from build123d import *

# Parameters (mm, degrees)
CROQUIS1_W              = 130
CROQUIS1_H              = 130
SALIENTE_EXTRUIR1_DEPTH = 60
REDONDEO1_R             = 10
VACIADO1_T              = -4
CORTAR_EXTRUIR1_START   = -58
CORTAR_EXTRUIR1_DEPTH   = 1
CORTAR_EXTRUIR2_START   = -56
CORTAR_EXTRUIR2_DEPTH   = 1
CORTAR_EXTRUIR3_START   = -4
CORTAR_EXTRUIR3_DEPTH   = 1


with BuildPart() as part:
    # Croquis1 → Saliente-Extruir1 (new body)
    with BuildSketch(Plane(origin=(0, 0, 0), x_dir=(1, 0, 0), z_dir=(0, 1, 0))):
        Rectangle(CROQUIS1_W, CROQUIS1_H)
    extrude(amount=SALIENTE_EXTRUIR1_DEPTH)

    # Redondeo1
    redondeo1_edges = [part.edges().sort_by_distance(p)[0] for p in [
        (-65, 30, -65),
        (65, 30, -65),
        (65, 30, 65),
        (-65, 30, 65),
    ]]
    fillet(redondeo1_edges, radius=REDONDEO1_R)

    # Vaciado1
    vaciado1_openings = [part.faces().sort_by_distance(p)[0] for p in [
        (0, 60, 0),
    ]]
    offset(amount=VACIADO1_T, openings=vaciado1_openings, kind=Kind.INTERSECTION)

    # Croquis2 → Cortar-Extruir1 (cut)
    with BuildSketch(Plane.XZ.offset(CORTAR_EXTRUIR1_START)):
        with BuildLine():
            Line((55, -65), (-55, -65))
            ThreePointArc((-55, -65), (-62.071067812, -62.071067812), (-65, -55))
            Line((-65, -55), (-65, 55))
            ThreePointArc((-65, 55), (-62.071067812, 62.071067812), (-55, 65))
            Line((-55, 65), (55, 65))
            ThreePointArc((55, 65), (62.071067812, 62.071067812), (65, 55))
            Line((65, 55), (65, -55))
            ThreePointArc((65, -55), (62.071067812, -62.071067812), (55, -65))
        make_face()
        with BuildLine():
            Line((55, -64.5), (-55, -64.5))
            ThreePointArc((-55, -64.5), (-61.717514421, -61.717514421), (-64.5, -55))
            Line((-64.5, -55), (-64.5, 55))
            ThreePointArc((-64.5, 55), (-61.717514421, 61.717514421), (-55, 64.5))
            Line((-55, 64.5), (55, 64.5))
            ThreePointArc((55, 64.5), (61.717514421, 61.717514421), (64.5, 55))
            Line((64.5, 55), (64.5, -55))
            ThreePointArc((64.5, -55), (61.717514421, -61.717514421), (55, -64.5))
        make_face(mode=Mode.SUBTRACT)
    extrude(amount=CORTAR_EXTRUIR1_DEPTH, mode=Mode.SUBTRACT)

    # Croquis2<2> → Cortar-Extruir2 (cut)
    with BuildSketch(Plane.XZ.offset(CORTAR_EXTRUIR2_START)):
        with BuildLine():
            Line((55, -65), (-55, -65))
            ThreePointArc((-55, -65), (-62.071067812, -62.071067812), (-65, -55))
            Line((-65, -55), (-65, 55))
            ThreePointArc((-65, 55), (-62.071067812, 62.071067812), (-55, 65))
            Line((-55, 65), (55, 65))
            ThreePointArc((55, 65), (62.071067812, 62.071067812), (65, 55))
            Line((65, 55), (65, -55))
            ThreePointArc((65, -55), (62.071067812, -62.071067812), (55, -65))
        make_face()
        with BuildLine():
            Line((55, -64.5), (-55, -64.5))
            ThreePointArc((-55, -64.5), (-61.717514421, -61.717514421), (-64.5, -55))
            Line((-64.5, -55), (-64.5, 55))
            ThreePointArc((-64.5, 55), (-61.717514421, 61.717514421), (-55, 64.5))
            Line((-55, 64.5), (55, 64.5))
            ThreePointArc((55, 64.5), (61.717514421, 61.717514421), (64.5, 55))
            Line((64.5, 55), (64.5, -55))
            ThreePointArc((64.5, -55), (61.717514421, -61.717514421), (55, -64.5))
        make_face(mode=Mode.SUBTRACT)
    extrude(amount=CORTAR_EXTRUIR2_DEPTH, mode=Mode.SUBTRACT)

    # Croquis2<3> → Cortar-Extruir3 (cut)
    with BuildSketch(Plane.XZ.offset(CORTAR_EXTRUIR3_START)):
        with BuildLine():
            Line((55, -65), (-55, -65))
            ThreePointArc((-55, -65), (-62.071067812, -62.071067812), (-65, -55))
            Line((-65, -55), (-65, 55))
            ThreePointArc((-65, 55), (-62.071067812, 62.071067812), (-55, 65))
            Line((-55, 65), (55, 65))
            ThreePointArc((55, 65), (62.071067812, 62.071067812), (65, 55))
            Line((65, 55), (65, -55))
            ThreePointArc((65, -55), (62.071067812, -62.071067812), (55, -65))
        make_face()
        with BuildLine():
            Line((55, -64.5), (-55, -64.5))
            ThreePointArc((-55, -64.5), (-61.717514421, -61.717514421), (-64.5, -55))
            Line((-64.5, -55), (-64.5, 55))
            ThreePointArc((-64.5, 55), (-61.717514421, 61.717514421), (-55, 64.5))
            Line((-55, 64.5), (55, 64.5))
            ThreePointArc((55, 64.5), (61.717514421, 61.717514421), (64.5, 55))
            Line((64.5, 55), (64.5, -55))
            ThreePointArc((64.5, -55), (61.717514421, -61.717514421), (55, -64.5))
        make_face(mode=Mode.SUBTRACT)
    extrude(amount=CORTAR_EXTRUIR3_DEPTH, mode=Mode.SUBTRACT)


solid = part.part
Here's how the part is built. I have some questions about the finished solid (model axes, mm). A direction names the side the tool comes from. Give positions to 0.01 mm unless a question says otherwise; leave off trailing zeros. Order: outer loops, then holes, each group sorted by start corner. A loop starts at its lowest first (then second) coordinate and runs counter-clockwise, first axis right, second up. Notation, with made-up numbers: (-23, 35) -> (10, 35) arc R34 ccw to (10, 72) -> close; hole circle Ø11 at (87, 9.25). An arc over 180 degrees is marked (long way). One line per item, written item: value. Start each with the question number.
1. Will these pins go through, and if not, where does the flat tip stop? pin 1 Ø8 at (x, z) = (32, -28) entering from +Y; pin 2 Ø0.5 at (y, z) = (55.5, -14) entering from +X; pin 3 Ø0.8 at (x, y) = (-20.5, 55.5) entering from +Z.
2. I need wall thicknesses on probe 1 along X at (y, z) = (42, 44); probe 2 along X at (y, z) = (55.5, 37). Which ranges of each line are inside material? Lowest first, please. Write a range as from..to.
3. Imagine slicing it at A-A, the plane y = 37. List the corners of the cut face in (x, z) for me, plus the area to 3 significant figures.
4. For faces 4 (the face through (61.791, 57.507, -61.643)), 5 (the face through (61.643, 3.507, 61.791)), 6 (the face through (-1, 32, -61)), 7 (the face through (-1, 29, -65)), 8 (the face through (-1, 0, -1)), which set-ups out of +Z, -Z, +X, -X, +Y, -Y let a thin tool reach every point of the face, with its end or its side?
5. We'd pull the mould along X, two halves only. Please class faces 1 (the face through (-62.15, 56.51, -61.99)), 2 (the face through (59.289, 32.392, -59.196)), 3 (the face through (61.791, 3.507, -61.643)): released by +X, released by -X, zero draft, split by the parting line, or undercut.
Values follow:
1. pin 1: stops at y = 4
1. pin 2: stops at x = 64.5
1. pin 3: stops at z = 64.5
2. probe 1: x = -65..-61, 61..65
2. probe 2: x = -64.5..-61, 61..64.5
3. outline: (-65, -55) arc R10 ccw to (-55, -65) -> (55, -65) arc R10 ccw to (65, -55) -> (65, 55) arc R10 ccw to (55, 65) -> (-55, 65) arc R10 ccw to (-65, 55) -> close; hole (-61, -55) arc R6 ccw to (-55, -61) -> (55, -61) arc R6 ccw to (61, -55) -> (61, 55) arc R6 ccw to (55, 61) -> (-55, 61) arc R6 ccw to (-61, 55) -> close
3. area: 1,960 mm2
4. face 4: -Z, +X
4. face 5: +Z, +X
4. face 6: +Y
4. face 7: -Z, +X, -X, +Y, -Y
4. face 8: +Z, -Z, +X, -X, -Y
5. face 1: released by -X
5. face 2: undercut
5. face 3: released by +X
